Can you work these out from the model? Positions are in its coordinate system, mm. A direction names the side the tool comes from. Round coordinates to 2 decimals unless told otherwise and drop trailing zeros. Order: outer loops, then holes, each group sorted by start corner. A loop starts at its lowest first (then second) coordinate and runs counter-clockwise, first axis right, second up. Notation, with made-up numbers: (85.25, -17) -> (109.25, -17) arc R25 cw to (109.25, 1) -> close; hole circle Ø5 at (-7, 27). An arc over 180 degrees is marked (long way). Use a Markdown table: item, result. Add a question column.
Q1. If we section it at C-C on x = 11: List the corners of the cut face in (y, z) for me.
Q2. I need wall thicknesses on line 1 along Y through (x, z) = (10.5, 1); line 2 along X through (y, z) = (7.75, 0.5); line 3 along X through (y, z) = (-6.5, 12.25). Which ranges of each line are inside material? Lowest first, please. Write a range as [from, to].
Q3. If we section it at A-A on x = 0: List the corners of the cut face in (y, z) for me, plus the area to 3 significant figures.
Q4. If we section it at B-B on y = -4: List the corners of the cut face in (x, z) for me.
Q5. For faces 5 (the face through (-9, 0, 8)), 6 (the face through (0, 6, -0.1)), 7 (the face through (0, -12, 0)), which set-ups out of +Z, -Z, +X, -X, +Y, -Y let a thin tool reach every point of the face, with its end or its side?
Q6. If we section it at D-D on z = 4.5: List the corners of the cut face in (x, y) for me.
Q7. We'd pull the mould along X, two halves only. Please class faces 1 (the face through (0.18, -8.25, 7.93)), 2 (the face through (0, 4, 3)), 3 (the face through (-13.75, 7, 1)), 4 (the face through (-12, 2, 1)): +X half, -X half, draft (parallel to the pull), parting line (faces both ways), or undercut.
Q8. I'm going to push flat-ended pins straight in: pin 1 Ø2 at (y, z) = (-7, 2.5) entering from +X; pin 2 Ø3.5 at (x, y) = (-2.5, 3) entering from -Z; pin 3 Ø6 at (x, y) = (4.5, 1.5) entering from +Z; pin 4 Ø6 at (y, z) = (7.5, 7.5) entering from -X. Where does each tip first touch, or does it pass through?
```python
from build123d import *

# Parameters (mm, degrees)
F1_DEPTH      = 1.8
F2_DEPTH      = 3
F2_DEPTH_BACK = 0.1
F3_DEPTH      = 13
F3_DEPTH_BACK = 1.7


with BuildPart() as f1:
    # F0 (on Top) → F1 (new body)
    with BuildSketch(Plane.XY):
        with BuildLine():
            Line((-13.75, 0), (-16.75, 0))
            ThreePointArc((-16.75, 0), (0, -16.75), (16.75, 0))
            Line((16.75, 0), (13.75, 0))
            Line((13.75, 0), (10.25, 0))
            ThreePointArc((10.25, 0), (0, -10.25), (-10.25, 0))
            Line((-10.25, 0), (-13.75, 0))
        make_face()
        with BuildLine():
            Line((-8.25, 0), (-10.25, 0))
            ThreePointArc((-10.25, 0), (0, -10.25), (10.25, 0))
            Line((10.25, 0), (8.25, 0))
            ThreePointArc((8.25, 0), (0, -8.25), (-8.25, 0))
        make_face()
        with BuildLine():
            Line((8.25, 0), (-8.25, 0))
            ThreePointArc((-8.25, 0), (0, -8.25), (8.25, 0))
        make_face()
    extrude(amount=-F1_DEPTH)

    # F0 (on Top) → F2 (join, two sides)
    with BuildSketch(Plane.XY) as f2_sk:
        with BuildLine():
            ThreePointArc((11.6859958925, 12), (12.7761141335, 10.8320546365), (13.75, 9.5655632349))
            Line((13.75, 9.5655632349), (13.75, 12))
            Line((13.75, 12), (11.6859958925, 12))
        make_face()
        with BuildLine():
            ThreePointArc((-10.0529846314, 2), (-10.2006272472, 1.0048401683), (-10.25, 0))
            Line((-10.25, 0), (-8.25, 0))
            ThreePointArc((-8.25, 0), (-8.1882451935, 1.0075418854), (-8.0039052968, 2))
            Line((-8.0039052968, 2), (-10.0529846314, 2))
        make_face()
        with BuildLine():
            ThreePointArc((-8.0039052968, 2), (-8.1882451935, 1.0075418854), (-8.25, 0))
            Line((-8.25, 0), (8.25, 0))
            ThreePointArc((8.25, 0), (8.1882451935, 1.0075418854), (8.0039052968, 2))
            Line((8.0039052968, 2), (-8.0039052968, 2))
        make_face()
        with BuildLine():
            Line((8.25, 0), (10.25, 0))
            ThreePointArc((10.25, 0), (10.2006272472, 1.0048401683), (10.0529846314, 2))
            Line((10.0529846314, 2), (8.0039052968, 2))
            ThreePointArc((8.0039052968, 2), (8.1882451935, 1.0075418854), (8.25, 0))
        make_face()
        with BuildLine():
            ThreePointArc((-11.6859958925, 12), (-12.7761141335, 10.8320546365), (-13.75, 9.5655632349))
            Line((-13.75, 9.5655632349), (-13.75, 2))
            Line((-13.75, 2), (-10.0529846314, 2))
            ThreePointArc((-10.0529846314, 2), (0, 10.25), (10.0529846314, 2))
            Line((10.0529846314, 2), (13.75, 2))
            Line((13.75, 2), (13.75, 9.5655632349))
            ThreePointArc((13.75, 9.5655632349), (12.7761141335, 10.8320546365), (11.6859958925, 12))
            Line((11.6859958925, 12), (-11.6859958925, 12))
        make_face()
        with BuildLine():
            Line((8.25, 0), (-8.25, 0))
            ThreePointArc((-8.25, 0), (0, -8.25), (8.25, 0))
        make_face()
        with BuildLine():
            Line((-8.25, 0), (-10.25, 0))
            ThreePointArc((-10.25, 0), (0, -10.25), (10.25, 0))
            Line((10.25, 0), (8.25, 0))
            ThreePointArc((8.25, 0), (0, -8.25), (-8.25, 0))
        make_face()
        with BuildLine():
            ThreePointArc((10.0529846314, 2), (0, 10.25), (-10.0529846314, 2))
            Line((-10.0529846314, 2), (-8.0039052968, 2))
            ThreePointArc((-8.0039052968, 2), (0, 8.25), (8.0039052968, 2))
            Line((8.0039052968, 2), (10.0529846314, 2))
        make_face()
        with BuildLine():
            ThreePointArc((8.0039052968, 2), (0, 8.25), (-8.0039052968, 2))
            Line((-8.0039052968, 2), (8.0039052968, 2))
        make_face()
        with BuildLine():
            Line((-13.75, 12), (-13.75, 9.5655632349))
            ThreePointArc((-13.75, 9.5655632349), (-12.7761141335, 10.8320546365), (-11.6859958925, 12))
            Line((-11.6859958925, 12), (-13.75, 12))
        make_face()
    extrude(amount=F2_DEPTH)
    extrude(f2_sk.sketch, amount=-F2_DEPTH_BACK)

    # F0 (on Top) → F3 (join, two sides)
    with BuildSketch(Plane.XY) as f3_sk:
        with BuildLine():
            Line((-8.25, 0), (-10.25, 0))
            ThreePointArc((-10.25, 0), (0, -10.25), (10.25, 0))
            Line((10.25, 0), (8.25, 0))
            ThreePointArc((8.25, 0), (0, -8.25), (-8.25, 0))
        make_face()
    extrude(amount=F3_DEPTH)
    extrude(f3_sk.sketch, amount=-F3_DEPTH_BACK)


solid = f1.part
```
Answer below:
| question | item | result |
|---|---|---|
| 1 | outline | (-12.63, -1.8) -> (0, -1.8) -> (0, 0) -> (-12.63, 0) -> close; (2, -0.1) -> (12, -0.1) -> (12, 3) -> (2, 3) -> close |
| 2 | line 1 | [2, 12] |
| 2 | line 2 | [-13.75, 13.75] |
| 2 | line 3 | [-7.93, -5.08], [5.08, 7.93] |
| 3 | outline | (-16.75, -1.8) -> (0, -1.8) -> (0, -0.1) -> (12, -0.1) -> (12, 3) -> (-8.25, 3) -> (-8.25, 13) -> (-10.25, 13) -> (-10.25, 0) -> (-16.75, 0) -> close |
| 3 | area | 118 mm² |
| 4 | outline | (-16.27, -1.8) -> (16.27, -1.8) -> (16.27, 0) -> (9.44, 0) -> (9.44, 13) -> (7.22, 13) -> (7.22, 3) -> (-7.22, 3) -> (-7.22, 13) -> (-9.44, 13) -> (-9.44, 0) -> (-16.27, 0) -> close |
| 5 | face 5 | +Z, +X, -X, +Y |
| 5 | face 6 | -Z, +X, -X, +Y |
| 5 | face 7 | +Z, -Y |
| 6 | outline | (-10.25, 0) arc R10.25 ccw to (10.25, 0) -> (8.25, 0) arc R8.25 cw to (-8.25, 0) -> close |
| 7 | face 1 | undercut |
| 7 | face 2 | undercut |
| 7 | face 3 | -X half |
| 7 | face 4 | draft |
| 8 | pin 1 | x = 8.31 |
| 8 | pin 2 | z = -0.1 |
| 8 | pin 3 | z = 3 |
| 8 | pin 4 | through |
